from build123d import *

# Parameters (mm, degrees)
SKETCH1_R           = 6.25
BOSS_EXTRUDE1_DEPTH = 2.5
SKETCH2_R           = 3.5
BOSS_EXTRUDE2_DEPTH = 6
CUT_EXTRUDE1_DEPTH  = 6


with BuildPart() as part:
    # Sketch1 → Boss-Extrude1 (new body)
    with BuildSketch(Plane(origin=(0, 0, 0), x_dir=(1, 0, 0), z_dir=(0, 1, 0))):
        with BuildLine():
            ThreePointArc((-5, 3.75), (0, 6.25), (5, 3.75))
            Line((5, 3.75), (2.75, 17.061179512))
            ThreePointArc((2.75, 17.061179512), (0, 19.385353712), (-2.75, 17.061179512))
            Line((-2.75, 17.061179512), (-5, 3.75))
        make_face()
        Circle(SKETCH1_R)
    extrude(amount=BOSS_EXTRUDE1_DEPTH)

    # Sketch2 → Boss-Extrude2 (add)
    with BuildSketch(Plane.XZ):
        with Locations(Location((0, 0, 0), (0, 0, 90))):
            Circle(SKETCH2_R)
    extrude(amount=BOSS_EXTRUDE2_DEPTH)

    # Sketch3 → Cut-Extrude1 (cut)
    with BuildSketch(Plane.XZ.offset(6)):
        with BuildLine():
            Line((-1.459451952, -1.475), (1.459451952, -1.475))
            ThreePointArc((1.459451952, -1.475), (1.91493966, -0.799143979), (2.075, 0))
            ThreePointArc((2.075, 0), (-0.799143979, 1.91493966), (-1.459451952, -1.475))
        make_face()
    extrude(amount=-CUT_EXTRUDE1_DEPTH, mode=Mode.SUBTRACT)


solid = part.part
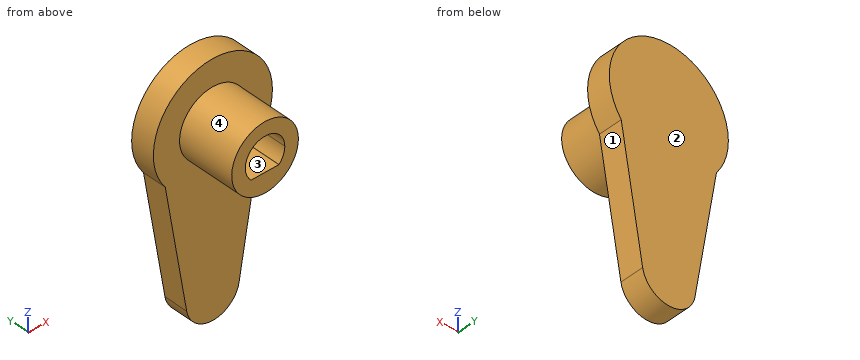
Verification items for the finished model (mm, model axes). Face numbers are marked on the shaded views. Coordinates: 2 decimals unless noted, no trailing zeros. Write each loop counter-clockwise with the first axis right and the second up, starting at its lowest first coordinate (ties: lowest second). Pieces come first, ordered by that corner, then holes. Notation, with made-up numbers: M 0.5,3 L 24.5,3 A13 ccw 24.5,19 Z; hole C 22.5,-28 d10. An arc over 180 degrees is marked long. Use CSV: the item, a comma, the result in double quotes.
Q1. Section check D-D, the plane y = 0.75. Enter the section's corners in (x, z), and give its area (3 significant figures).
Computed values:
outline,"M -5,-3.75 L -2.75,-17.06 A2.79 ccw 2.75,-17.06 L 5,-3.75 A6.25 ccw long Z"
area,"218 mm²"
Q2. Section check A-A, the plane x = 0. Enter the section's corners in (y, z) (3 decimals).
Computed values:
outline,"M -6,-3.5 L 0,-3.5 L 0,-19.385 L 2.5,-19.385 L 2.5,6.25 L 0,6.25 L 0,3.5 L -6,3.5 L -6,2.075 L 0,2.075 L 0,-1.475 L -6,-1.475 Z"
Q3. Mould release check, pull along X, two halves, no side actions. Record for the marked faces 1, 2, 3 and 4: pulls with the +X half, pulls with the -X half, needs draft (parallel to the pull), parting line crosses it, or undercut.
Computed values:
face 1,"pulls with the +X half"
face 2,"needs draft"
face 3,"undercut"
face 4,"parting line crosses it"
Q4. Thickness scan on line 1 along X through (y, z) = (-2.4, 0) (3 decimals); line 2 along Y through (x, z) = (1.25, 0); line 3 along Z through (x, y) = (0.5, -3.75) (3 decimals). Record the ranges inside material, lowest first. Write a range as [from, to].
Computed values:
line 1,"[-3.5, -2.075], [2.075, 3.5]"
line 2,"[0, 2.5]"
line 3,"[-3.464, -1.475], [2.014, 3.464]"
Q5. Go/stop test with flat-tipped pins: P1, Ø4, axis at x = -3, y = -1.5, coming from the +Z side; P2, Ø1.5, axis at y = 0, z = -2.5, coming from the +X side; P3, Ø1.8, axis at x = -0.5, z = 0, coming from the -Y side. Record where each tip stops, or that it passes through.
Computed values:
P1,"z = 6.02"
P2,"x = 6"
P3,"y = 0"
Q6. Section check C-C, the plane y = -1.5. Enter the section's corners in (x, z) (3 decimals).
Computed values:
outline,"C 0,0 d7; hole M -1.459,-1.475 L 1.459,-1.475 A2.075 ccw long Z"
Q7. Section check B-B, the plane z = -1.75. Enter the section's corners in (x, y).
Computed values:
outline,"M -6,0 L -3.03,0 L -3.03,-6 L 3.03,-6 L 3.03,0 L 6,0 L 6,2.5 L -6,2.5 Z"
